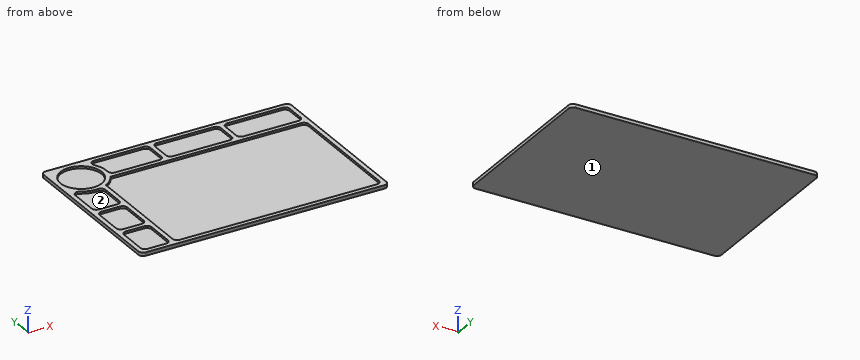
```python
from build123d import *

# Parameters (mm, degrees)
F0_W     = 30
F0_H     = 40
F0_R     = 22.5
F0_W_2   = 70
F0_H_2   = 30
F1_DEPTH = 3.7
F2_DEPTH = 1.3
F3_R     = 5


with BuildPart() as f1:
    # F0 (on Top) → F1 (new body)
    with BuildSketch(Plane.XY):
        with BuildLine():
            Line((129.123384, 121.491298), (-130.876616, 121.491298))
            ThreePointArc((-130.876616, 121.491298), (-134.41215, 120.026832), (-135.876616, 116.491298))
            Line((-135.876616, 116.491298), (-135.876616, -58.508702))
            ThreePointArc((-135.876616, -58.508702), (-134.41215, -62.044236), (-130.876616, -63.508702))
            Line((-130.876616, -63.508702), (129.123384, -63.508702))
            ThreePointArc((129.123384, -63.508702), (132.658918, -62.044236), (134.123384, -58.508702))
            Line((134.123384, -58.508702), (134.123384, 116.491298))
            ThreePointArc((134.123384, 116.491298), (132.658918, 120.026832), (129.123384, 121.491298))
        make_face()
        with Locations((-115.876616, -38.508702)):
            Rectangle(F0_W, F0_H, mode=Mode.SUBTRACT)
        with Locations((-115.876616, 6.491298)):
            Rectangle(F0_W, F0_H, mode=Mode.SUBTRACT)
        with BuildLine():
            ThreePointArc((-95.876616, 69.4964), (-88.93118, 74.545861), (-83.881719, 81.491298))
            Line((-83.881719, 81.491298), (129.123384, 81.491298))
            Line((129.123384, 81.491298), (129.123384, -58.508702))
            Line((129.123384, -58.508702), (-95.876616, -58.508702))
            Line((-95.876616, -58.508702), (-95.876616, 69.4964))
        make_face(mode=Mode.SUBTRACT)
        with BuildLine():
            Line((-130.876616, 31.491298), (-130.876616, 78.179909))
            ThreePointArc((-130.876616, 78.179909), (-117.573626, 68.074797), (-100.876616, 67.533784))
            Line((-100.876616, 67.533784), (-100.876616, 31.491298))
            Line((-100.876616, 31.491298), (-130.876616, 31.491298))
        make_face(mode=Mode.SUBTRACT)
        with Locations((-108.376616, 93.991298)):
            Circle(F0_R, mode=Mode.SUBTRACT)
        with BuildLine():
            Line((-23.623535, 86.491298), (-81.919103, 86.491298))
            ThreePointArc((-81.919103, 86.491298), (-82.460116, 103.188308), (-92.565228, 116.491298))
            Line((-92.565228, 116.491298), (-23.623535, 116.491298))
            Line((-23.623535, 116.491298), (-22.565228, 116.491298))
            Line((-22.565228, 116.491298), (-22.565228, 86.491298))
            Line((-22.565228, 86.491298), (-23.623535, 86.491298))
        make_face(mode=Mode.SUBTRACT)
        Polygon((54.123384, 86.491298), (12.149697, 86.491298), (-17.565228, 86.491298), (-17.565228, 116.491298), (54.123384, 116.491298), align=None, mode=Mode.SUBTRACT)
        with Locations((94.123384, 101.491298)):
            Rectangle(F0_W_2, F0_H_2, mode=Mode.SUBTRACT)
    extrude(amount=F1_DEPTH)

    # F0 (on Top) → F2 (join)
    with BuildSketch(Plane.XY):
        with BuildLine():
            Line((129.123384, 121.491298), (-130.876616, 121.491298))
            ThreePointArc((-130.876616, 121.491298), (-134.41215, 120.026832), (-135.876616, 116.491298))
            Line((-135.876616, 116.491298), (-135.876616, -58.508702))
            ThreePointArc((-135.876616, -58.508702), (-134.41215, -62.044236), (-130.876616, -63.508702))
            Line((-130.876616, -63.508702), (129.123384, -63.508702))
            ThreePointArc((129.123384, -63.508702), (132.658918, -62.044236), (134.123384, -58.508702))
            Line((134.123384, -58.508702), (134.123384, 116.491298))
            ThreePointArc((134.123384, 116.491298), (132.658918, 120.026832), (129.123384, 121.491298))
        make_face()
        with Locations((-115.876616, -38.508702)):
            Rectangle(F0_W, F0_H, mode=Mode.SUBTRACT)
        with Locations((-115.876616, 6.491298)):
            Rectangle(F0_W, F0_H, mode=Mode.SUBTRACT)
        with BuildLine():
            ThreePointArc((-95.876616, 69.4964), (-88.93118, 74.545861), (-83.881719, 81.491298))
            Line((-83.881719, 81.491298), (129.123384, 81.491298))
            Line((129.123384, 81.491298), (129.123384, -58.508702))
            Line((129.123384, -58.508702), (-95.876616, -58.508702))
            Line((-95.876616, -58.508702), (-95.876616, 69.4964))
        make_face(mode=Mode.SUBTRACT)
        with BuildLine():
            Line((-130.876616, 31.491298), (-130.876616, 78.179909))
            ThreePointArc((-130.876616, 78.179909), (-117.573626, 68.074797), (-100.876616, 67.533784))
            Line((-100.876616, 67.533784), (-100.876616, 31.491298))
            Line((-100.876616, 31.491298), (-130.876616, 31.491298))
        make_face(mode=Mode.SUBTRACT)
        with Locations((-108.376616, 93.991298)):
            Circle(F0_R, mode=Mode.SUBTRACT)
        with BuildLine():
            Line((-23.623535, 86.491298), (-81.919103, 86.491298))
            ThreePointArc((-81.919103, 86.491298), (-82.460116, 103.188308), (-92.565228, 116.491298))
            Line((-92.565228, 116.491298), (-23.623535, 116.491298))
            Line((-23.623535, 116.491298), (-22.565228, 116.491298))
            Line((-22.565228, 116.491298), (-22.565228, 86.491298))
            Line((-22.565228, 86.491298), (-23.623535, 86.491298))
        make_face(mode=Mode.SUBTRACT)
        Polygon((54.123384, 86.491298), (12.149697, 86.491298), (-17.565228, 86.491298), (-17.565228, 116.491298), (54.123384, 116.491298), align=None, mode=Mode.SUBTRACT)
        with Locations((94.123384, 101.491298)):
            Rectangle(F0_W_2, F0_H_2, mode=Mode.SUBTRACT)
        with BuildLine():
            Line((129.123384, 81.491298), (-83.881719, 81.491298))
            ThreePointArc((-83.881719, 81.491298), (-88.93118, 74.545861), (-95.876616, 69.4964))
            Line((-95.876616, 69.4964), (-95.876616, -58.508702))
            Line((-95.876616, -58.508702), (129.123384, -58.508702))
            Line((129.123384, -58.508702), (129.123384, 81.491298))
        make_face()
        with Locations((94.123384, 101.491298)):
            Rectangle(F0_W_2, F0_H_2)
        Polygon((-17.565228, 86.491298), (12.149697, 86.491298), (54.123384, 86.491298), (54.123384, 116.491298), (-17.565228, 116.491298), align=None)
        with BuildLine():
            ThreePointArc((-92.565228, 116.491298), (-82.460116, 103.188308), (-81.919103, 86.491298))
            Line((-81.919103, 86.491298), (-23.623535, 86.491298))
            Line((-23.623535, 86.491298), (-22.565228, 86.491298))
            Line((-22.565228, 86.491298), (-22.565228, 116.491298))
            Line((-22.565228, 116.491298), (-23.623535, 116.491298))
            Line((-23.623535, 116.491298), (-92.565228, 116.491298))
        make_face()
        with Locations((-108.376616, 93.991298)):
            Circle(F0_R)
        with BuildLine():
            ThreePointArc((-100.876616, 67.533784), (-117.573626, 68.074797), (-130.876616, 78.179909))
            Line((-130.876616, 78.179909), (-130.876616, 31.491298))
            Line((-130.876616, 31.491298), (-100.876616, 31.491298))
            Line((-100.876616, 31.491298), (-100.876616, 67.533784))
        make_face()
        with Locations((-115.876616, 6.491298)):
            Rectangle(F0_W, F0_H)
        with Locations((-115.876616, -38.508702)):
            Rectangle(F0_W, F0_H)
    extrude(amount=F2_DEPTH)

    # F3
    f3_edges = [f1.edges().sort_by_distance(p)[0] for p in [
        (59.123384, 116.491298, 2.5),
        (129.123384, 81.491298, 2.5),
        (129.123384, 116.491298, 2.5),
        (129.123384, 86.491298, 2.5),
        (59.123384, 86.491298, 2.5),
        (54.123384, 86.491298, 2.5),
        (54.123384, 116.491298, 2.5),
        (-17.565228, 86.491298, 2.5),
        (-81.919103, 86.491298, 2.5),
        (-130.876616, -13.508702, 2.5),
        (-100.876616, 26.491298, 2.5),
        (-100.876616, 67.533784, 2.5),
        (-100.876616, -18.508702, 2.5),
        (-130.876616, 26.491298, 2.5),
        (-130.876616, 78.179909, 2.5),
        (-92.565228, 116.491298, 2.5),
        (-17.565228, 116.491298, 2.5),
        (-130.876616, -58.508702, 2.5),
        (-130.876616, 31.491298, 2.5),
        (-100.876616, -13.508702, 2.5),
        (-100.876616, 31.491298, 2.5),
        (-100.876616, -58.508702, 2.5),
        (-95.876616, -58.508702, 2.5),
        (-130.876616, -18.508702, 2.5),
        (129.123384, -58.508702, 2.5),
        (-22.565228, 86.491298, 2.5),
        (-22.565228, 116.491298, 2.5),
    ]]
    fillet(f3_edges, radius=F3_R)


solid = f1.part
```
Part model, mm, in its own coordinate system. Face numbers are marked on the shaded views. Coordinates: 2 decimals unless noted, no trailing zeros. Order: outer loops, then holes, each group sorted by start corner. A loop starts at its lowest first (then second) coordinate and runs counter-clockwise, first axis right, second up. Notation, with made-up numbers: (10.5, -31) -> (31.5, -31) arc R21 cw to (31.5, -11) -> close; hole circle Ø8 at (-31, 46). An arc over 180 degrees is marked (long way). Put each result on its own line as item: value. Start each with the question number.
(1) Mould opens along Z. For the marked faces 1 and 2 say: pulls with the +Z half, pulls with the -Z half, needs draft (parallel to the pull), parting line crosses it, or undercut.
(2) Probe line 1 along X through (y, z) = (-46.5, 2); line 2 along Y through (x, z) = (44.5, 3.35); line 3 along Y through (x, z) = (-117, 2). List the from-to ranges inside material, lowest first. Write a range as [from, to].
(3) Pin check, flat tip, straight feed: pin 1 Ø8 at (x, y) = (9, 91) entering from +Z. Stop position of the tip, or through.
(4) Band-saw the part on B-B (y = -40.5). Give the cut face in (x, z), then the cut area to 3 significant figures.
(5) Band-saw the part on A-A (x = 105). Give the cut face in (y, z), then the cut area to 4 significant figures.
Determined:
1. face 1: pulls with the -Z half
1. face 2: pulls with the +Z half
2. line 1: x = [-135.88, -130.88], [-100.88, -95.88], [129.12, 134.12]
2. line 2: y = [-63.51, -58.51], [81.49, 86.49], [116.49, 121.49]
2. line 3: y = [-63.51, -58.51], [-18.51, -13.51], [26.49, 31.49], [67.88, 73.21], [114.77, 121.49]
3. pin 1: stops at z = 1.3
4. outline: (-135.88, 0) -> (134.12, 0) -> (134.12, 3.7) -> (129.12, 3.7) -> (129.12, 1.3) -> (-95.88, 1.3) -> (-95.88, 3.7) -> (-100.88, 3.7) -> (-100.88, 1.3) -> (-130.88, 1.3) -> (-130.88, 3.7) -> (-135.88, 3.7) -> close
4. area: 387 mm²
5. outline: (-63.51, 0) -> (121.49, 0) -> (121.49, 3.7) -> (116.49, 3.7) -> (116.49, 1.3) -> (86.49, 1.3) -> (86.49, 3.7) -> (81.49, 3.7) -> (81.49, 1.3) -> (-58.51, 1.3) -> (-58.51, 3.7) -> (-63.51, 3.7) -> close
5. area: 276.5 mm²
